Work out the finished part from the listing and answer in its coordinate system (mm). Round coordinates to 2 decimals unless told otherwise and drop trailing zeros. Order: outer loops, then holes, each group sorted by start corner. A loop starts at its lowest first (then second) coordinate and runs counter-clockwise, first axis right, second up. Notation, with made-up numbers: M 67.5,89.5 L 126.5,89.5 A3 cw 126.5,93.5 Z; hole C -6.75,50 d5. An arc over 180 degrees is marked long. Return JSON: item names as keys, results as strings.
from build123d import *

# Parameters (mm, degrees)
BOSS_EXTRUDE1_DEPTH   = 3.81
F_4_40_TAPPED_HOLE1_D = 1.7526
CUT_EXTRUDE1_DEPTH    = 25.948437705


with BuildPart() as part:
    # Sketch1 → Boss-Extrude1 (new body)
    with BuildSketch(Plane(origin=(0, 0, 0), x_dir=(1, 0, 0), z_dir=(0, 1, 0))):
        with BuildLine():
            Line((0.307655172, 6.517241379), (0.307655172, -18.882758621))
            ThreePointArc((0.307655172, -18.882758621), (4.498655172, -23.073758621), (8.689655172, -18.882758621))
            Line((8.689655172, -18.882758621), (8.689655172, 6.517241379))
            ThreePointArc((8.689655172, 6.517241379), (4.498655172, 10.708241379), (0.307655172, 6.517241379))
        make_face()
    extrude(amount=BOSS_EXTRUDE1_DEPTH)

    # #4-40 Tapped Hole1 (through all)
    with Locations(Plane(origin=(0, 3.81, 0), x_dir=(1, 0, 0), z_dir=(0, 1, 0))):
        with Locations((4.498655172, 6.517241379), (4.498655172, -18.882758621)):
            Hole(F_4_40_TAPPED_HOLE1_D / 2)

    # Sketch4 → Cut-Extrude1 (cut, through all)
    with BuildSketch(Plane(origin=(0, 3.81, 0), x_dir=(1, 0, 0), z_dir=(0, 1, 0))):
        with BuildLine():
            Line((0.307655172, -17.084100697), (0.307655172, -1.885416544))
            ThreePointArc((0.307655172, -1.885416544), (1.807655172, -9.484758621), (0.307655172, -17.084100697))
        make_face()
    extrude(amount=-CUT_EXTRUDE1_DEPTH, mode=Mode.SUBTRACT)


solid = part.part
Item 1: Consider line 1 along X through (y, z) = (3.6, 19); line 2 along Z through (x, y) = (5, 1.5); line 3 along Z through (x, y) = (4.25, 0.6). Determine where each line is inside the solid, lowest interval first. Write a range as [from, to].
Output:
{"line 1": "x = [0.31, 3.63], [5.37, 8.69]", "line 2": "z = [-10.68, -7.24], [-5.8, 18.16], [19.6, 23.04]", "line 3": "z = [-10.7, -7.36], [-5.68, 18.04], [19.72, 23.07]"}
Item 2: Each of these flat-tipped pins is pushed along its axis until it touches: pin 1 (1.6 mm diameter, centred on x = 4.5, z = -6.52, fed in from -Y); pin 2 (1.5 mm diameter, centred on y = 2.5, z = 8, fed in from -X); pin 3 (1 mm diameter, centred on x = 6.5, y = 0.5, fed in from +Z). Where does it stop, or does it pass through?
Output:
{"pin 1": "passes through", "pin 2": "stops at x = 1.68", "pin 3": "stops at z = 22.8"}
Item 3: Find section D-D (z = 12.5). Determine the outline of the cut face in (x, y), plus the area to 3 significant figures.
Output:
{"outline": "M 1.58,0 L 8.69,0 L 8.69,3.81 L 1.58,3.81 Z", "area": "27.1 mm^2"}
Item 4: The mould has two halves that part along Z. Classify faces 1 (the cylindrical face through (4.689, 1.878, 19.738)), 2 (the cylindrical face through (4.406, 1.878, 23.073)), 3 (the cylindrical face through (4.613, 1.878, -7.386)), 4 (the flat face through (4, 0, 6)): pulls with the +Z half, pulls with the -Z half, needs draft (parallel to the pull), parting line crosses it, or undercut.
Output:
{"face 1": "undercut", "face 2": "pulls with the +Z half", "face 3": "undercut", "face 4": "needs draft"}
Item 5: Find section C-C (z = -6). Determine the outline of the cut face in (x, y).
Output:
{"outline": "M 0.31,0 L 3.79,0 L 3.79,3.81 L 0.31,3.81 Z; M 5.21,0 L 8.69,0 L 8.69,3.81 L 5.21,3.81 Z"}
Item 6: Find section B-B (x = 4.5). Determine the outline of the cut face in (y, z).
Output:
{"outline": "M 0,-10.71 L 3.81,-10.71 L 3.81,-7.39 L 0,-7.39 Z; M 0,-5.64 L 3.81,-5.64 L 3.81,18.01 L 0,18.01 Z; M 0,19.76 L 3.81,19.76 L 3.81,23.07 L 0,23.07 Z"}
Item 7: Find section A-A (y = 0.95). Determine the outline of the cut face in (x, z), plus the area to 3 significant figures.
Output:
{"outline": "M 0.31,-6.52 A4.19 ccw 8.69,-6.52 L 8.69,18.88 A4.19 ccw 0.31,18.88 L 0.31,17.08 A20 cw 0.31,1.89 Z; hole C 4.5,-6.52 d1.75; hole C 4.5,18.88 d1.75", "area": "248 mm^2"}
